from build123d import *

# Parameters (mm, degrees)
F0_R     = 10
F1_DEPTH = 2.5
F2_R     = 10
F2_R_2   = 8.5
F3_DEPTH = 3
F4_R     = 2.5
F5_DEPTH = 4


with BuildPart() as f1:
    # F0 (on Top) → F1 (new body, symmetric)
    with BuildSketch(Plane.XY):
        Circle(F0_R)
    extrude(amount=F1_DEPTH, both=True)

    # F2 (on face) → F3 (cut)
    with BuildSketch(Plane.XY.offset(2.5)):
        Circle(F2_R)
        Circle(F2_R_2, mode=Mode.SUBTRACT)
    extrude(amount=-F3_DEPTH, mode=Mode.SUBTRACT)

    # F4 (on face) → F5 (cut)
    with BuildSketch(Plane(origin=(0, 0, -2.5), x_dir=(1, 0, 0), z_dir=(0, 0, -1))):
        Circle(F4_R)
    extrude(amount=-F5_DEPTH, mode=Mode.SUBTRACT)


solid = f1.part
For this review, take the finished solid that the model builds, in its own axes (mm). A direction names the side the tool comes from. Coordinates: 2 decimals unless noted, no trailing zeros. Order: outer loops, then holes, each group sorted by start corner. A loop starts at its lowest first (then second) coordinate and runs counter-clockwise, first axis right, second up. Notation, with made-up numbers: (18, -16) -> (27, -16) arc R35 ccw to (27, 17) -> close; hole circle Ø11 at (21.25, -22). An arc over 180 degrees is marked (long way). Return JSON: item names as keys, results as strings.
1. For pin 1 Ø1.5 at (x, y) = (0, -1) entering from -Z; pin 2 Ø2 at (x, y) = (-0.5, 1.5) entering from -Z; pin 3 Ø2 at (x, z) = (4, 2) entering from +Y; pin 4 Ø1.5 at (y, z) = (-5, 1.5) entering from -X, all flat-tipped, find the tip position at first contact; note any pin that passes through.
Answer block:
{"pin 1": "z = 1.5", "pin 2": "z = -2.5", "pin 3": "y = 7.95", "pin 4": "x = -7.36"}
2. For line 1 (Y direction, x = 0, z = -1.1); line 2 (Z direction, x = -7.75, y = 4.25); line 3 (X direction, y = -2, z = -1.45), list the stretches that pass through material, from the lowest coordinate up. Write a range as from..to.
Answer block:
{"line 1": "-10..-2.5, 2.5..10", "line 2": "-2.5..-0.5", "line 3": "-9.8..-1.5, 1.5..9.8"}
3. We need section C-C on z = -1.7. Write out the cut boundary in (x, y).
Answer block:
{"outline": "circle Ø20 at (0, 0); hole circle Ø5 at (0, 0)"}
4. We need section A-A on x = 0. Write out the cut boundary in (y, z).
Answer block:
{"outline": "(-10, -2.5) -> (-2.5, -2.5) -> (-2.5, 1.5) -> (2.5, 1.5) -> (2.5, -2.5) -> (10, -2.5) -> (10, -0.5) -> (8.5, -0.5) -> (8.5, 2.5) -> (-8.5, 2.5) -> (-8.5, -0.5) -> (-10, -0.5) -> close"}
5. The part is to be moulded in two halves that separate along X. For faces 3 (the flat face through (0, 0, 1.5)), 4 (the flat face through (-4.5, -7.4, -0.5)), 5 (the cylindrical face through (4.57, 7.167, 1.021)), say which applies: +X half, -X half, draft (parallel to the pull), parting line (faces both ways), or undercut.
Answer block:
{"face 3": "undercut", "face 4": "draft", "face 5": "parting line"}
6. Machinability: for faces 1 (the flat face through (0, 0, 2.5)), 2 (the cylindrical face through (-0.54, 2.44, -0.53)), which of the approach directions +Z, -Z, +X, -X, +Y, -Y give a long, thin tool a straight path to every point of the face, cutting with its end or side? Answer none if there is none.
Answer block:
{"face 1": "+Z, +X, -X, +Y, -Y", "face 2": "-Z"}
7. We need section D-D on z = 2.2. Write out the cut boundary in (x, y).
Answer block:
{"outline": "circle Ø17 at (0, 0)"}
